Input: part model. Units: mm. Frame: model coordinates. A direction names the side the tool comes from. Give positions to 0.01 mm unless a question says otherwise; leave off trailing zeros. Write each loop counter-clockwise with the first axis right and the second up, starting at its lowest first coordinate (ties: lowest second). Pieces come first, ordered by that corner, then holes. Notation, with made-up numbers: (87, 44) -> (100, 44) arc R12 ccw to (100, 55) -> close; hole circle Ø10 at (-36.75, 8). An arc over 180 degrees is marked (long way). Return JSON: item names as keys, results as strings. Group by question number.
Item 1: Line query: line 1 (X direction, y = 18, z = -63); line 2 (Y direction, x = 106.45, z = -45); line 3 (Z direction, x = 51.5, y = 14). Output: solid intervals per line, ascending. Write a range as [from, to].
Item 2: Section C-C, the plane x = 66. Return loops of the section in (y, z), then the cut area to 3 significant figures.
Item 3: Mould query, pull axis X, two halves, no side actions, for faces 5 (the face through (13, -13, 27)), 6 (the face through (2.528, 2.379, 42.253)), 7 (the face through (0, 3, -1)). Classes: released by +X, released by -X, zero draft, split by the parting line, or undercut.
Item 4: Section D-D, the plane y = 9.5. Return loops of the section in (x, z).
Item 5: Section A-A, the plane z = 26.5. Return loops of the section in (x, y), then the cut area to 3 significant figures.
Item 6: Section B-B, the plane z = -45. Return loops of the section in (x, y).
Item 7: Pin query (flat end, axial travel): P1, Ø8.5, axis at x = 78, z = -22, coming from the +Y side; P2, Ø1, axis at x = 77, y = 1, coming from the +Z side; P3, Ø1.5, axis at x = 70.5, y = -12.5, coming from the +Z side. Return the tip coordinate at first contact, or that it passes through.
Item 8: Set-up query: faces 1 (the face through (5, 7, 42)), 2 (the face through (54, -10, -14)), 3 (the face through (55, -13, 20)), 4 (the face through (13, -13, -27)). Return all of +Z, -Z, +X, -X, +Y, -Y with unobstructed straight access to the full face (end or side cutting, diameter ignored); none if empty.
from build123d import *

# Parameters (mm, degrees)
SKETCH_1_W          = 160
SKETCH_1_H          = 20
EXTRUDE_1_DEPTH     = 5
EXTRUDE_3_DEPTH     = 100
SKETCH_5_W          = 12
SKETCH_5_H          = 15
EXTRUDE_4_DEPTH     = 105
SKETCH_6_W          = 74
SKETCH_6_H          = 15
EXTRUDE_5_DEPTH     = 5
SKETCH_7_W          = 160
SKETCH_7_H          = 35
EXTRUDE_6_DEPTH     = 5
EXTRUDE_7_DEPTH     = 5
SKETCH_9_R          = 2.75
CUT_EXTRUDE_1_DEPTH = 138.477270849
CHAMFER_1_SIZE      = 0.5
FILLET_1_R          = 10


with BuildPart() as part:
    # 草图1 → 凸台-拉伸1 (new body)
    with BuildSketch(Plane(origin=(0, 0, 0), x_dir=(0, 0, -1), z_dir=(1, 0, 0))):
        with Locations((0, -5)):
            Rectangle(SKETCH_1_W, SKETCH_1_H)
    extrude(amount=EXTRUDE_1_DEPTH)

    # 草图3 → 凸台-拉伸3 (add)
    with BuildSketch(Plane(origin=(5, 0, 0), x_dir=(0, 0, -1), z_dir=(1, 0, 0))):
        Polygon((-6, 5), (6, 5), (6, -10), (20, -10), (20, -15), (-20, -15), (-20, -10), (-6, -10), align=None)
    extrude(amount=EXTRUDE_3_DEPTH)

    # 草图5 → 凸台-拉伸4 (add)
    with BuildSketch(Plane.ZY):
        with Locations((0, 12.5)):
            Rectangle(SKETCH_5_W, SKETCH_5_H)
    extrude(amount=-EXTRUDE_4_DEPTH)

    # 草图6 → 凸台-拉伸5 (add)
    with BuildSketch(Plane.ZY):
        with Locations((43, 12.5)):
            Rectangle(SKETCH_6_W, SKETCH_6_H)
        with Locations((-43, 12.5)):
            Rectangle(SKETCH_6_W, SKETCH_6_H)
    extrude(amount=-EXTRUDE_5_DEPTH)

    # 草图7 → 凸台-拉伸6 (add)
    with BuildSketch(Plane(origin=(105, 0, 0), x_dir=(0, 0, -1), z_dir=(1, 0, 0))):
        with Locations((0, 2.5)):
            Rectangle(SKETCH_7_W, SKETCH_7_H)
    extrude(amount=EXTRUDE_6_DEPTH)

    # 草图8 → 凸台-拉伸7 (add)
    with BuildSketch(Plane.XZ.offset(15)):
        Polygon((90, 20), (105, 35), (105, 20), align=None)
        Polygon((105, -20), (90, -20), (105, -35), align=None)
        Polygon((5, 20), (20, 20), (5, 35), align=None)
        Polygon((20, -20), (5, -35), (5, -20), align=None)
    extrude(amount=-EXTRUDE_7_DEPTH)

    # 草图9 → 切除-拉伸1 (cut, through all)
    with BuildSketch(Plane(origin=(110, 0, 0), x_dir=(0, 0, -1), z_dir=(1, 0, 0))):
        with Locations((45, 2.5)):
            Circle(SKETCH_9_R)
        with Locations(Location((-45, 2.5, 0), (0, 0, 180))):
            Circle(SKETCH_9_R)
    extrude(amount=-CUT_EXTRUDE_1_DEPTH, mode=Mode.SUBTRACT)

    # 倒角1
    chamfer_1_edges = [part.edges().sort_by_distance(p)[0] for p in [
        (105, 2.5, -42.25),
        (5, 2.5, -42.25),
        (0, 2.5, -42.25),
        (110, 2.5, -42.25),
        (105, 2.5, 42.25),
        (5, 2.5, 42.25),
        (0, 2.5, 42.25),
        (110, 2.5, 42.25),
    ]]
    chamfer(chamfer_1_edges, length=CHAMFER_1_SIZE)

    # 圆角1
    fillet_1_edges = [part.edges().sort_by_distance(p)[0] for p in [
        (107.5, -15, 80),
        (107.5, -15, -80),
        (2.5, -15, -80),
        (2.5, -15, 80),
    ]]
    fillet(fillet_1_edges, radius=FILLET_1_R)


solid = part.part
Answer below:
{
 "1": {"line 1": "x = [0, 5], [105, 110]", "line 2": "y = [-15, -0.25], [5.25, 20]", "line 3": "z = [-6, 6]"},
 "2": {"outline": "(-15, -20) -> (-10, -20) -> (-10, -6) -> (20, -6) -> (20, 6) -> (-10, 6) -> (-10, 20) -> (-15, 20) -> close", "area": "560 mm2"},
 "3": {"face 5": "undercut", "face 6": "zero draft", "face 7": "released by -X"},
 "4": {"outline": "(0, -80) -> (5, -80) -> (5, -6) -> (105, -6) -> (105, -80) -> (110, -80) -> (110, 80) -> (105, 80) -> (105, 6) -> (5, 6) -> (5, 80) -> (0, 80) -> close"},
 "5": {"outline": "(0, -15) -> (13.5, -15) -> (13.5, -10) -> (5, -10) -> (5, 20) -> (0, 20) -> close; (96.5, -15) -> (110, -15) -> (110, 20) -> (105, 20) -> (105, -10) -> (96.5, -10) -> close", "area": "435 mm2"},
 "6": {"outline": "(0, -15) -> (5, -15) -> (5, -0.75) -> (4.5, -0.25) -> (0.5, -0.25) -> (0, -0.75) -> close; (0, 5.75) -> (0.5, 5.25) -> (4.5, 5.25) -> (5, 5.75) -> (5, 20) -> (0, 20) -> close; (105, -15) -> (110, -15) -> (110, -0.75) -> (109.5, -0.25) -> (105.5, -0.25) -> (105, -0.75) -> close; (105, 5.75) -> (105.5, 5.25) -> (109.5, 5.25) -> (110, 5.75) -> (110, 20) -> (105, 20) -> close"},
 "7": {"P1": "stops at y = -10", "P2": "stops at z = 6", "P3": "stops at z = 20"},
 "8": {"face 1": "+Z, +Y", "face 2": "-Z, +Y", "face 3": "+Z, +Y, -Y", "face 4": "-Z, +Y, -Y"}
}
